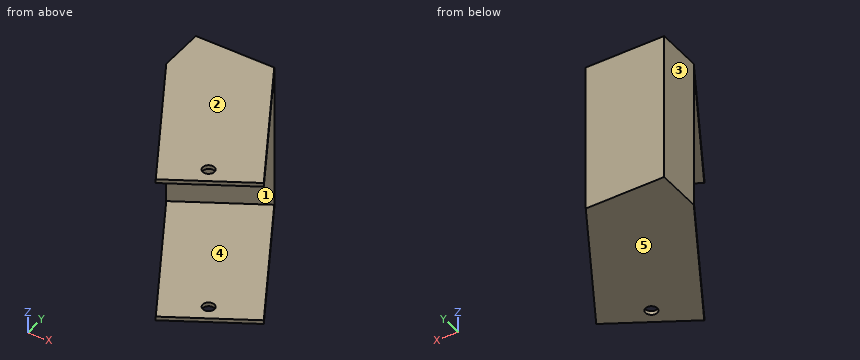
```python
from build123d import *

# Parameters (mm, degrees)
F1_DEPTH = 60.325
F3_DEPTH = 3.175
F5_DEPTH = 3.175
F6_R     = 4.7625
F7_DEPTH = 120.651


with BuildPart() as f1:
    # F0 (on Top) → F1 (new body, symmetric)
    with BuildSketch(Plane.XY):
        Polygon((63.241505, 0), (0, 0), (0, -36.5125), align=None)
    extrude(amount=F1_DEPTH, both=True)

    # F2 (on face) → F3 (join)
    with BuildSketch(Plane.XY.offset(60.325)):
        Polygon((63.241505, 0), (0, -36.5125), (63.5, -146.497726), (126.741505, -109.985226), align=None)
    extrude(amount=-F3_DEPTH)

    # F4 (on face) → F5 (join)
    with BuildSketch(Plane(origin=(0, 0, -60.325), x_dir=(1, 0, 0), z_dir=(0, 0, -1))):
        Polygon((63.5, 146.497726), (0, 36.5125), (63.241505, 0), (126.741505, 109.985226), align=None)
    extrude(amount=-F5_DEPTH)

    # F6 (on face) → F7 (cut, through all)
    with BuildSketch(Plane.XY.offset(60.325)):
        with Locations((87.504892, -117.973799)):
            Circle(F6_R)
    extrude(amount=-F7_DEPTH, mode=Mode.SUBTRACT)


solid = f1.part
```
Here's how the part is built. I have some questions about the finished solid (model axes, mm). Face numbers are marked on the shaded views. A direction names the side the tool comes from. Give positions to 0.01 mm unless a question says otherwise; leave off trailing zeros. Order: outer loops, then holes, each group sorted by start corner. A loop starts at its lowest first (then second) coordinate and runs counter-clockwise, first axis right, second up. Notation, with made-up numbers: M 45.25,13 L 53.25,13 A21 ccw 53.25,34 Z; hole C 24,34 d6. An arc over 180 degrees is marked long. Use a Markdown table: item, result. Add a question column.
1. I need wall thicknesses on probe 1 along Z at (x, y) = (93, -116) (3 decimals); probe 2 along Y at (x, z) = (12, -24); probe 3 along X at (y, z) = (-7.5, 51.5). Which ranges of each line are inside material? Lowest first, please. Write a range as from..to.
2. Suppose I cut it at A-A (y = -74.5). List the corners of the cut face in (x, z) for me (3 decimals), and give its area (3 significant figures).
3. Suppose I cut it at D-D (y = -9). List the corners of the cut face in (x, z) for me (3 decimals), and give its area (3 significant figures).
4. On a 3-axis mill with a long thin cutter (end or side, diameter ignored), from which of +Z, -Z, +X, -X, +Y, -Y can I reach the whole of each face in a straight line? I mean the marked faces 1 and 2. Say none if no direction works.
5. If we mould it in two halves opening along Z, with no side actions, what happens to the marked faces 3, 4 and 5? For each: +Z half, -Z half, draft (parallel to the pull), parting line (faces both ways), or undercut.
6. Suppose I cut it at B-B (x = 104.5). List the corners of the cut face in (y, z) for me (3 decimals).
7. For pin 1 Ø5.5 at (x, y) = (87.5, -117.97) entering from -Z, with a flat end and sliding along its axis, tell me the tip position at first contact or that it passes through.
8. Suppose I cut it at C-C (x = 23). List the corners of the cut face in (y, z) for me (3 decimals), and give its area (3 significant figures).
Results list:
| question | item | result |
|---|---|---|
| 1 | probe 1 | z = -60.325..-57.15, 57.15..60.325 |
| 1 | probe 2 | y = -29.58..0 |
| 1 | probe 3 | x = 0..50.25 |
| 2 | outline | M 21.932,-60.325 L 106.254,-60.325 L 106.254,-57.15 L 21.932,-57.15 Z; M 21.932,57.15 L 106.254,57.15 L 106.254,60.325 L 21.932,60.325 Z |
| 2 | area | 535 mm² |
| 3 | outline | M 0,-60.325 L 68.438,-60.325 L 68.438,-57.15 L 47.653,-57.15 L 47.653,57.15 L 68.438,57.15 L 68.438,60.325 L 0,60.325 Z |
| 3 | area | 5,880 mm² |
| 4 | face 1 | +X, -Y |
| 4 | face 2 | +Z, +X, -X, +Y, -Y |
| 5 | face 3 | draft |
| 5 | face 4 | undercut |
| 5 | face 5 | -Z half |
| 6 | outline | M -122.826,-60.325 L -71.462,-60.325 L -71.462,-57.15 L -122.826,-57.15 Z; M -122.826,57.15 L -71.462,57.15 L -71.462,60.325 L -122.826,60.325 Z |
| 7 | pin 1 | passes through |
| 8 | outline | M -76.35,-60.325 L 0,-60.325 L 0,60.325 L -76.35,60.325 L -76.35,57.15 L -23.233,57.15 L -23.233,-57.15 L -76.35,-57.15 Z |
| 8 | area | 3,140 mm² |
